Check sheet for the modelled part. Datum: model origin and axes. Units: mm. A direction names the side the tool comes from. Round coordinates to 2 decimals unless told otherwise and drop trailing zeros. Order: outer loops, then holes, each group sorted by start corner. A loop starts at its lowest first (then second) coordinate and runs counter-clockwise, first axis right, second up. Notation, with made-up numbers: (-34.75, -13) -> (8.25, -13) arc R17 ccw to (8.25, 13) -> close; hole circle Ø9 at (23.25, 55). An arc over 180 degrees is marked (long way). Use CSV: the item, a comma, the result in double quotes.
Autodesk Inventor part; units mm, degrees
ref_plane "YZ Plane" through (0, 0, 0) normal (1, 0, 0) x (0, 1, 0)
ref_plane "XZ Plane" through (0, 0, 0) normal (0, 1, 0) x (-1, 0, 0)
ref_plane "XY Plane" through (0, 0, 0) normal (0, 0, 1) x (1, 0, 0)
sketch "スケッチ1" plane through (0, 0, 0) normal (0, 0, 1) x (1, 0, 0)
  line L0 (29, -43.5) -> (-29, -43.5)
  line L1 (-29, -43.5) -> (-29, 43.5)
  line L2 (-29, 43.5) -> (29, 43.5)
  line L3 (29, 43.5) -> (29, -43.5)
  line L4 (29, -43.5) -> (-29, 43.5) construction
  line L5 (-29, -43.5) -> (29, 43.5) construction
  point P0 (0, 0)
  dimension "d0" = 87
  dimension "d1" = 58
extrude "プレート1" add sketch "スケッチ1" along normal blind 3
sketch "スケッチ2" plane through (-32, 43.5, -3) normal (-1, 0, 0) x (0, -1, 0)
  line L0 (87, 0) -> (0, 0)
  line L1 (0, 0) -> (0, -16)
  line L2 (0, -16) -> (87, -16)
  line L3 (87, -16) -> (87, 0)
edge flange "フランジ1" height 22 angle 90 thickness 3 bend radius 3 thickness toward (-1, 0, 0) relief tear relief width 3 relief depth 1.5 edges at (-29, 0, 0) wall of the first edge with corners at (-32, -43.5, -3) (-32, 43.5, -3) (-32, 43.5, -19) (-32, -43.5, -19)
bend "曲げ1"
corner "コーナー1"
sketch "スケッチ3" plane through (29, 46.5, -3) normal (0, 1, 0) x (-1, 0, 0)
  line L0 (58, 0) -> (0, 0)
  line L1 (0, 0) -> (0, -16)
  line L2 (0, -16) -> (58, -16)
  line L3 (58, -16) -> (58, 0)
edge flange "フランジ2" height 22 angle 90 thickness 3 bend radius 3 thickness toward (0, 1, 0) relief tear relief width 3 relief depth 1.5 edges at (0, 43.5, 0) wall of the first edge with corners at (-29, 46.5, -3) (29, 46.5, -3) (29, 46.5, -19) (-29, 46.5, -19)
bend "曲げ2"
corner "コーナー2"
sketch "スケッチ4" plane through (0, 0, 3) normal (0, 0, 1) x (1, 0, 0)
  line L0 (29, -43.5) -> (-29, -43.5)
  line L1 (-24, -43.5) -> (33.3099, 38.5)
  line L2 (-29, -43.5) -> (-29, 43.5)
  line L3 (-29, 43.5) -> (29, 43.5)
  line L4 (-29, -43.5) -> (-29, 43.5)
  line L5 (29, -43.5) -> (-29, -43.5)
  line L6 (29, 43.5) -> (29, -43.5)
  line L7 (-29, 43.5) -> (29, 43.5)
  point P0 (0, 0)
  point P1 (29, 32.3333)
  dimension "d23" = 5
  dimension "d24" = 5
extrude "押し出し1" cut sketch "スケッチ4" against normal through all contours L0 L1 L6
fillet "フィレット1" radius 2 6 edges at (-24, -43.5, 1.5) (-33.5, -43.5, -19) (29, 32.3333, 1.5) (29, 48, -19) (-33.5, 43.5, -19) (-29, 48, -19)
sketch "スケッチ5" plane through (-32, -43.5, -3) normal (1, 0, 0) x (0, 0, -1)
  arc A0 (16, 85) -> (14, 87) centre (14, 85) ccw
  line L0 (14, 87) -> (0, 87)
  line L1 (0, 87) -> (0, 0)
  line L2 (14, 0) -> (0, 0)
  arc A1 (14, 0) -> (16, 2) centre (14, 2) ccw
  line L3 (16, 2) -> (16, 85)
  point P0 (-3, 43.5)
  point P1 (8, 77)
  point P2 (8, 10)
  point P3 (8, 43.5)
  dimension "d28" = 8
  dimension "d29" = 10
  dimension "d30" = 10
  dimension "d31" = 33.5
hole "穴1" at (-32, 33.5, -11) at (-32, -33.5, -11) at (-32, 0, -11) direction (-1, 0, 0) diameter 3.242 end through all
sketch "スケッチ6" plane through (-29, 49.5, -3) normal (0, 1, 0) x (1, 0, 0)
  line L0 (10, 8) -> (48, 8)
  line L1 (2, 16) -> (56, 16)
  line L2 (58, 14) -> (58, 0)
  line L3 (0, 0) -> (0, 14)
  point P0 (29, -3)
  point P1 (29, 8)
  dimension "d39" = 8
  dimension "d40" = 10
  dimension "d41" = 10
hole "穴2" at (0, 49.5, -11) at (19, 49.5, -11) at (-19, 49.5, -11) direction (0, -1, 0) diameter 3.242 end through all
sketch "スケッチ8" plane through (0, 0, 3) normal (0, 0, 1) x (1, 0, 0)
  line L0 (-29, 49.5) -> (29, 49.5)
  line L1 (29, 43.5) -> (29, 32.9629)
  point P0 (0, 0)
  point P1 (9, 37.5)
  dimension "d54" = 12
  dimension "d55" = 20
hole "穴3" at (9, 37.5, 3) direction (0, 0, -1) diameter 8.2 end through all
equation "\"d61\" = Thickness"
equation "\"d2\" = Thickness"
equation "\"d3\" = BendReliefWidth"
equation "\"d4\" = BendReliefDepth"
equation "\"d5\" = MinimumRemnant"
equation "\"d6\" = TransitionRadius"
equation "\"d9\" = BendRadius"
equation "\"d10\" = CornerReliefSize"
equation "\"d11\" = GapSize"
equation "\"d12\" = JacobiRadiusSize"
equation "\"d13\" = BendReliefWidth"
equation "\"d14\" = BendReliefDepth"
equation "\"d15\" = MinimumRemnant"
equation "\"d16\" = TransitionRadius"
equation "\"d19\" = BendRadius"
equation "\"d20\" = CornerReliefSize"
equation "\"d21\" = GapSize"
equation "\"d22\" = JacobiRadiusSize"
equation "\"BendRadius\" = Thickness"
equation "\"BendReliefWidth\" = Thickness"
equation "\"BendReliefDepth\" = 0.5 * Thickness"
equation "\"CornerReliefSize\" = 4 * Thickness"
equation "\"MinimumRemnant\" = 2 * Thickness"
equation "\"TransitionRadius\" = BendRadius"
equation "\"JacobiRadiusSize\" = BendRadius"
equation "\"GapSize\" = Thickness"
properties part number "CCM_Mount_C"
Q1. Sectioned sample at D-D, the plane x = -22. Enter the section's corners in (y, z), then the cut area to 3 significant figures.
Result sheet:
outline,"(-40.64, 0) -> (43.5, 0) arc R3 cw to (46.5, -3) -> (46.5, -19) -> (49.5, -19) -> (49.5, -3) arc R6 ccw to (43.5, 3) -> (-40.64, 3) -> close"
area,"322 mm^2"
Q2. Scan lines: L1, parallel to X at y = 48.25, z = -11; L2, parallel to Y at x = -34.2, z = -11; L3, parallel to Z at x = -32.8, y = 33.5. Record each from-to range of solid material in increasing order.
Result sheet:
L1,"x = -29 to -20.62, -17.38 to -1.62, 1.62 to 17.38, 20.62 to 29"
L2,"y = -43.5 to -35.12, -31.88 to -1.62, 1.62 to 31.88, 35.12 to 43.5"
L3,"z = -19 to -12.62, -9.38 to 1.64"
Q3. Mould release check, pull along Z, two halves, no side actions. Record for faces 3 (the face through (-7, 10, 3)), 4 (the face through (-29, 47, -7)), 5 (the face through (-33.521, -31.918, -10.649)): pulls with the +Z half, pulls with the -Z half, needs draft (parallel to the pull), parting line crosses it, or undercut.
Result sheet:
face 3,"pulls with the +Z half"
face 4,"needs draft"
face 5,"undercut"
Q4. Sectioned sample at C-C, the plane x = 9. Enter the section's corners in (y, z).
Result sheet:
outline,"(3.72, 0) -> (33.4, 0) -> (33.4, 3) -> (3.72, 3) -> close; (41.6, 0) -> (43.5, 0) arc R3 cw to (46.5, -3) -> (46.5, -19) -> (49.5, -19) -> (49.5, -3) arc R6 ccw to (43.5, 3) -> (41.6, 3) -> close"
Q5. Sectioned sample at B-B, the plane z = -11. State how many separate pieces and enclosed holes the cut face has, then the cut area to 3 significant figures.
Result sheet:
separate pieces,"8"
enclosed holes,"0"
area,"377 mm^2"
Q6. Sectioned sample at A-A, the plane y = 37.5. Enter the section's corners in (x, z).
Result sheet:
outline,"(-35, -19) -> (-32, -19) -> (-32, -3) arc R3 cw to (-29, 0) -> (4.9, 0) -> (4.9, 3) -> (-29, 3) arc R6 ccw to (-35, -3) -> close; (13.1, 0) -> (29, 0) -> (29, 3) -> (13.1, 3) -> close"
Q7. Access from +Z, -Z, +X, -X, +Y, -Y to the whole of each face (thin tool, end or side, straight path). Record for faces 1 (the face through (-7, 10, 0)), 2 (the face through (-33, 1, -19)).
Result sheet:
face 1,"-Z, +X, -Y"
face 2,"-Z, +X, -X, +Y, -Y"
Q8. Go/stop test with flat-tipped pins: pin 1 (10 mm diameter, centred on x = -20.5, z = -4, fed in from -Y); pin 2 (1 mm diameter, centred on x = -19, z = -1, fed in from -Y); pin 3 (13 mm diameter, centred on y = 0.5, z = -8, fed in from +X). Record where each tip stops, or that it passes through.
Result sheet:
pin 1,"stops at y = -42.77"
pin 2,"stops at y = 45.16"
pin 3,"stops at x = -31.6"
